Part model, mm, in its own coordinate system. Give positions to 0.01 mm unless a question says otherwise; leave off trailing zeros. Write each loop counter-clockwise with the first axis right and the second up, starting at its lowest first coordinate (ties: lowest second). Pieces come first, ordered by that corner, then holes.
```python
from build123d import *

# Parameters (mm, degrees)
BOSS_EXTRUDE1_DEPTH = 1


with BuildPart() as part:
    # Sketch1 → Boss-Extrude1 (new body)
    with BuildSketch(Plane(origin=(40.721862841, -259.93142883, 0), x_dir=(0.987949588, 0.154776003, 0), z_dir=(0.154776003, -0.987949588, 0))):
        Polygon((2498.917023581, -58.444774641), (2498.917023581, -139.900786314), (2074.988000168, -194.317166252), (2074.988000168, 194.317166252), (2498.917023581, 139.900786314), (2498.917023581, 58.444774641), align=None)
        with BuildLine():
            Line((2473.917023581, -58.444774641), (2473.917023581, -112.625661461))
            ThreePointArc((2473.917023581, -112.625661461), (2472.421655996, -116.589029575), (2468.680927979, -118.57683362))
            Line((2468.680927979, -118.57683362), (2106.751904566, -165.034769173))
            ThreePointArc((2106.751904566, -165.034769173), (2102.024632054, -163.588229428), (2099.988000168, -159.083597013))
            Line((2099.988000168, -159.083597013), (2099.988000168, 159.083597013))
            ThreePointArc((2099.988000168, 159.083597013), (2102.024632054, 163.588229428), (2106.751904566, 165.034769173))
            Line((2106.751904566, 165.034769173), (2468.680927979, 118.57683362))
            ThreePointArc((2468.680927979, 118.57683362), (2472.421655996, 116.589029575), (2473.917023581, 112.625661461))
            Line((2473.917023581, 112.625661461), (2473.917023581, 58.444774641))
            Line((2473.917023581, 58.444774641), (2473.917023581, -58.444774641))
        make_face(mode=Mode.SUBTRACT)
    extrude(amount=BOSS_EXTRUDE1_DEPTH)


solid = part.part
```
1) Pin check, flat tips, straight feed: pin 1 Ø12 at (x, y) = (2221.5, 76) entering from -Z; pin 2 Ø10 at (x, y) = (2240, 85) entering from +Z. Stop position of each tip, or through.
Answers follow:
pin 1: stops at z = -177.92
pin 2: stops at z = 175.55
2) Saw through at B-B, the plane y = 101. Write the cut outline in (x, z).
Answers follow:
outline: (2344.58, -161.33) - (2351.04, -160.51) - (2351.04, -135.31) - (2344.58, -136.13) - close; (2344.58, 136.13) - (2351.04, 135.31) - (2351.04, 160.51) - (2344.58, 161.33) - close
3) Wall check: L1, parallel to Y at x = 2237, z = 169; L2, parallel to Y at x = 2184, z = -171. Give the ranges that are in metal, low to high.
Answers follow:
L1: y = 83.13 to 84.15
L2: y = 74.83 to 75.84
4) Saw through at A-A, the plane z = -74. Write the cut outline in (x, y).
Answers follow:
outline: (2090.71, 61.23) - (2090.86, 60.24) - (2115.56, 64.11) - (2115.4, 65.1) - close; (2484.83, 122.97) - (2484.98, 121.98) - (2509.68, 125.85) - (2509.53, 126.84) - close
